Design review of the part built by this model. Coordinates are the model's own, in mm. Coordinates: 2 decimals unless noted, no trailing zeros. Write each loop counter-clockwise with the first axis right and the second up, starting at its lowest first coordinate (ties: lowest second). Pieces come first, ordered by that corner, then holes. Notation, with made-up numbers: M -34,17.5 L 20,17.5 A19 ccw 20,33.5 Z; hole C 23,81 d2. An arc over 180 degrees is marked long. Write item = value, one per line.
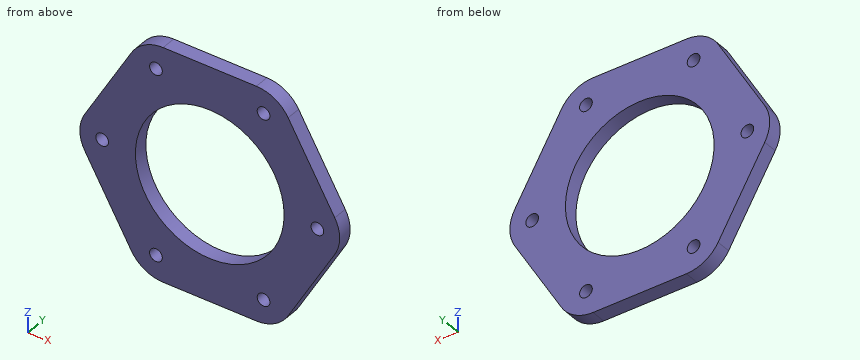
```python
from build123d import *

# Parameters (mm, degrees)
F0_R     = 2.6
F0_R_2   = 30.4
F1_DEPTH = 6
F2_R     = 15


with BuildPart() as f1:
    # F0 (on Front) → F1 (new body)
    with BuildSketch(Plane.XZ):
        Polygon((27.712813, 48), (-27.712813, 48), (-55.425626, 0), (-27.712813, -48), (27.712813, -48), (55.425626, 0), align=None)
        with Locations((-22, -38.105118)):
            Circle(F0_R, mode=Mode.SUBTRACT)
        with Locations((-44, 0)):
            Circle(F0_R, mode=Mode.SUBTRACT)
        Circle(F0_R_2, mode=Mode.SUBTRACT)
        with Locations((22, -38.105118)):
            Circle(F0_R, mode=Mode.SUBTRACT)
        with Locations((44, 0)):
            Circle(F0_R, mode=Mode.SUBTRACT)
        with Locations((-22, 38.105118)):
            Circle(F0_R, mode=Mode.SUBTRACT)
        with Locations((22, 38.105118)):
            Circle(F0_R, mode=Mode.SUBTRACT)
    extrude(amount=F1_DEPTH)

    # F2
    f2_edges = [f1.edges().sort_by_distance(p)[0] for p in [
        (-27.712813, -3, 48),
        (-55.425626, -3, 0),
        (-27.712813, -3, -48),
        (27.712813, -3, -48),
        (55.425626, -3, 0),
        (27.712813, -3, 48),
    ]]
    fillet(f2_edges, radius=F2_R)


solid = f1.part
```
Q1. Consider section A-A, the plane z = 0. State the section outline as (x, y) points.
Check result:
outline = M -53.11,-6 L -46.6,-6 L -46.6,0 L -53.11,0 Z; M -41.4,-6 L -30.4,-6 L -30.4,0 L -41.4,0 Z; M 30.4,-6 L 41.4,-6 L 41.4,0 L 30.4,0 Z; M 46.6,-6 L 53.11,-6 L 53.11,0 L 46.6,0 Z
Q2. Wall thickness on line 1 (Z direction, x = 0, y = -2.8); line 2 (X direction, y = -3.6, z = -36); line 3 (X direction, y = -5.45, z = -1.5): over which ranges is each line inside the solid? List them lowest first.
Check result:
line_1 = -48 to -30.4, 30.4 to 48
line_2 = -34.64 to -23.53, -20.47 to 20.47, 23.53 to 34.64
line_3 = -53.03 to -46.12, -41.88 to -30.36, 30.36 to 41.88, 46.12 to 53.03
Q3. Consider section C-C, the plane y = -3.3. State the section outline as (x, z) points.
Check result:
outline = M -51.1,-7.5 L -32.04,-40.5 A15 ccw -19.05,-48 L 19.05,-48 A15 ccw 32.04,-40.5 L 51.1,-7.5 A15 ccw 51.1,7.5 L 32.04,40.5 A15 ccw 19.05,48 L -19.05,48 A15 ccw -32.04,40.5 L -51.1,7.5 A15 ccw Z; hole C -44,0 d5.2; hole C 0,0 d60.8; hole C -22,-38.11 d5.2; hole C -22,38.11 d5.2; hole C 22,-38.11 d5.2; hole C 22,38.11 d5.2; hole C 44,0 d5.2
Q4. For P1, Ø1, axis at y = -1.5, z = -11, coming from the -X side; P2, Ø4.5, axis at x = -22, z = -38.11, coming from the -Y side, all flat-tipped, find the tip position at first contact; note any pin that passes through.
Check result:
P1 = -49.36
P2 = through
Q5. Consider section B-B, the plane x = 0. State the section outline as (y, z) points, and give its area (3 significant figures).
Check result:
outline = M -6,-48 L 0,-48 L 0,-30.4 L -6,-30.4 Z; M -6,30.4 L 0,30.4 L 0,48 L -6,48 Z
area = 211 mm²
Q6. Consider section D-D, the plane x = 22. State the section outline as (y, z) points.
Check result:
outline = M -6,-47.71 L 0,-47.71 L 0,-40.71 L -6,-40.71 Z; M -6,-35.51 L 0,-35.51 L 0,-20.98 L -6,-20.98 Z; M -6,20.98 L 0,20.98 L 0,35.51 L -6,35.51 Z; M -6,40.71 L 0,40.71 L 0,47.71 L -6,47.71 Z
